For this review, take the finished solid that the model builds, in its own axes (mm). Face numbers are marked on the shaded views. A direction names the side the tool comes from. Give positions to 0.01 mm unless a question says otherwise; leave off trailing zeros. Write each loop counter-clockwise with the first axis right and the second up, starting at its lowest first coordinate (ties: lowest second). Pieces come first, ordered by that corner, then holes. Notation, with made-up numbers: (67.25, 21.25) -> (119.25, 21.25) arc R24 ccw to (119.25, 32.25) -> close; hole circle Ø3 at (12, 66.5). An arc over 180 degrees is marked (long way). Return JSON: item names as keys, results as strings.
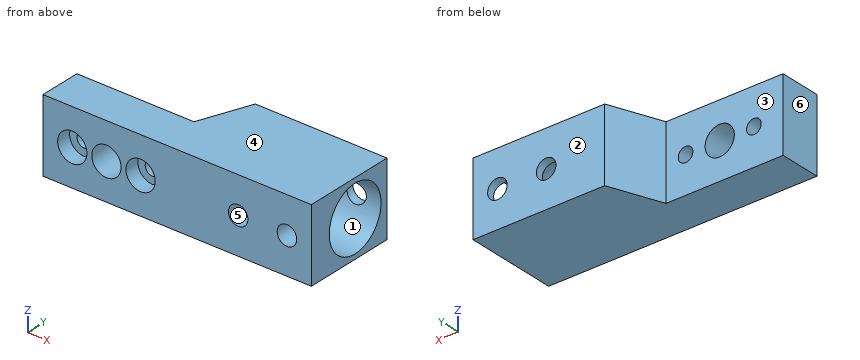
from build123d import *

# Parameters (mm, degrees)
SKETCH1_W               = 15
SKETCH1_H               = 19
SKETCH1_R               = 6.5
BOSS_EXTRUDE1_DEPTH     = 25
SKETCH2_W               = 15
SKETCH2_H               = 19
BOSS_EXTRUDE2_DEPTH     = 2
CUT_EXTRUDE1_DEPTH      = 29.324018077
CUT_EXTRUDE1_DEPTH_BACK = 29.324018077
SKETCH4_R               = 2
SKETCH3_W               = 28
SKETCH3_H               = 15
SKETCH3_R               = 3
BOSS_EXTRUDE3_DEPTH     = 8.5
CHAMFER1_SIZE2          = 10.5
CHAMFER1_SIZE           = 4
SKETCH6_R               = 1.5
CUT_EXTRUDE3_DEPTH      = 33.657311618
SKETCH7_R               = 3
CUT_EXTRUDE4_DEPTH      = 3


with BuildPart() as part:
    # Sketch1 → Boss-Extrude1 (new body)
    with BuildSketch(Plane(origin=(0, 0, 0), x_dir=(0, 0, -1), z_dir=(1, 0, 0))):
        with Locations((0, -1.5)):
            Rectangle(SKETCH1_W, SKETCH1_H)
        Circle(SKETCH1_R, mode=Mode.SUBTRACT)
    extrude(amount=BOSS_EXTRUDE1_DEPTH)

    # Sketch2 → Boss-Extrude2 (add)
    with BuildSketch(Plane(origin=(0, 0, 0), x_dir=(0, 0, -1), z_dir=(1, 0, 0))):
        with Locations((0, -1.5)):
            Rectangle(SKETCH2_W, SKETCH2_H)
    extrude(amount=-BOSS_EXTRUDE2_DEPTH)

    # Sketch4 → Cut-Extrude1 (cut, two sides: drawn at the far end of the back side and taken through both)
    with BuildSketch(Plane(origin=(0, 0, 0), x_dir=(1, 0, 0), z_dir=(0, 1, 0)).offset(-CUT_EXTRUDE1_DEPTH_BACK)):
        with Locations(Location((10, 0, 0), (0, 0, 270))):
            Circle(SKETCH4_R)
        with Locations(Location((20, 0, 0), (0, 0, 270))):
            Circle(SKETCH4_R)
    extrude(amount=CUT_EXTRUDE1_DEPTH + CUT_EXTRUDE1_DEPTH_BACK, mode=Mode.SUBTRACT)

    # Sketch3 → Boss-Extrude3 (add)
    with BuildSketch(Plane(origin=(0, -2.5, 0), x_dir=(1, 0, 0), z_dir=(0, 1, 0))):
        with Locations((-16, 0)):
            Rectangle(SKETCH3_W, SKETCH3_H)
        with Locations(Location((-17, 0, 0), (0, 0, 270))):
            Circle(SKETCH3_R, mode=Mode.SUBTRACT)
    extrude(amount=-BOSS_EXTRUDE3_DEPTH)

    # Chamfer1
    chamfer1_edges = [part.edges().sort_by_distance(p)[0] for p in [
        (-2, -2.5, 0),
    ]]
    chamfer1_side = [part.faces().sort_by_distance(p)[0] for p in [
        (-2.08, -2.5, 0),
    ]]
    chamfer(chamfer1_edges, length=CHAMFER1_SIZE - 0.0001, length2=CHAMFER1_SIZE2 - 0.0001, reference=chamfer1_side[0])  # a hair under: the kernel refuses the full size

    # Sketch6 → Cut-Extrude3 (cut, through all)
    with BuildSketch(Plane(origin=(0, -2.5, 0), x_dir=(1, 0, 0), z_dir=(0, 1, 0))):
        with Locations(Location((-24, 0, 0), (0, 0, 270))):
            Circle(SKETCH6_R)
        with Locations(Location((-10, 0, 0), (0, 0, 270))):
            Circle(SKETCH6_R)
    extrude(amount=-CUT_EXTRUDE3_DEPTH, mode=Mode.SUBTRACT)

    # Sketch7 → Cut-Extrude4 (cut)
    with BuildSketch(Plane.XZ.offset(11)):
        with Locations(Location((-10, 0, 0), (0, 0, 270))):
            Circle(SKETCH7_R)
        with Locations(Location((-24, 0, 0), (0, 0, 90))):
            Circle(SKETCH7_R)
    extrude(amount=-CUT_EXTRUDE4_DEPTH, mode=Mode.SUBTRACT)


solid = part.part
1. Add section A-A, the plane x = -24. State the section outline as (y, z) points, plus the area to 3 significant figures.
Results found:
{"outline": "(-11, -7.5) -> (-2.5, -7.5) -> (-2.5, -1.5) -> (-8, -1.5) -> (-8, -3) -> (-11, -3) -> close; (-11, 3) -> (-8, 3) -> (-8, 1.5) -> (-2.5, 1.5) -> (-2.5, 7.5) -> (-11, 7.5) -> close", "area": "93.0 mm²"}
2. For pin 1 (5 mm diameter, centred on x = -17, z = 0, fed in from +Y); pin 2 (4 mm diameter, centred on x = -10, z = 0, fed in from -Y); pin 3 (3 mm diameter, centred on y = 2.5, z = -4, fed in from -X), all flat-tipped, find the tip position at first contact; note any pin that passes through.
Results found:
{"pin 1": "passes through", "pin 2": "stops at y = -8", "pin 3": "stops at x = -4.67"}
3. The part is to be moulded in two halves that separate along Z. For the marked faces 4, 5 and 6, say which applies: +Z half, -Z half, draft (parallel to the pull), parting line (faces both ways), or undercut.
Results found:
{"face 4": "+Z half", "face 5": "undercut", "face 6": "draft"}
4. For the marked faces 1, 2 and 3, list the 3-axis set-ups (+Z, -Z, +X, -X, +Y, -Y) from which the entire face can be reached by the end or side of a thin tool; tool diameter is ignored.
Results found:
{"face 1": "+X", "face 2": "+Z, -Z, +X, -X, +Y", "face 3": "+Z, -Z, -X, +Y"}
5. Add section D-D, the plane x = 17. State the section outline as (y, z) points.
Results found:
{"outline": "(-11, -7.5) -> (8, -7.5) -> (8, 7.5) -> (-11, 7.5) -> close; hole circle Ø13 at (0, 0)"}
6. Add section C-C, the plane x = -17. State the section outline as (y, z) points.
Results found:
{"outline": "(-11, -7.5) -> (-2.5, -7.5) -> (-2.5, -3) -> (-11, -3) -> close; (-11, 3) -> (-2.5, 3) -> (-2.5, 7.5) -> (-11, 7.5) -> close"}
7. Add section B-B, the plane z = 0. Count the separate pieces of the cut face and the enclosed holes in it, plus the area to 3 significant figures.
Results found:
{"separate pieces": "8", "enclosed holes": "0", "area": "279 mm²"}
8. To check wall thickness, follow probe 1 along X at (y, z) = (-7.5, 0); probe 2 along X at (y, z) = (-10, 0); probe 3 along X at (y, z) = (-4.5, 0). State the ranges of each line that lie inside material, in increasing order.
Results found:
{"probe 1": "x = -30 to -25.5, -22.5 to -20, -14 to -11.5, -8.5 to 8, 12 to 18, 22 to 25", "probe 2": "x = -30 to -27, -21 to -20, -14 to -13, -7 to 8, 12 to 18, 22 to 25", "probe 3": "x = -30 to -25.5, -22.5 to -20, -14 to -11.5, -8.5 to 0"}
